Design review of the part built by this model. Coordinates are the model's own, in mm. Face numbers are marked on the shaded views. A direction names the side the tool comes from. Give positions to 0.01 mm unless a question says otherwise; leave off trailing zeros. Loops run counter-clockwise (first coordinate to the right, second up) from the corner with the lowest first, then second, coordinate; pieces in that order, holes last. Notation, with made-up numbers: M 88.25,44 L 106.25,44 A28 cw 106.25,73 Z; hole C 65.5,29.25 d11. An arc over 180 degrees is marked long. Use one line per item in the form item = value. Start each with the question number.
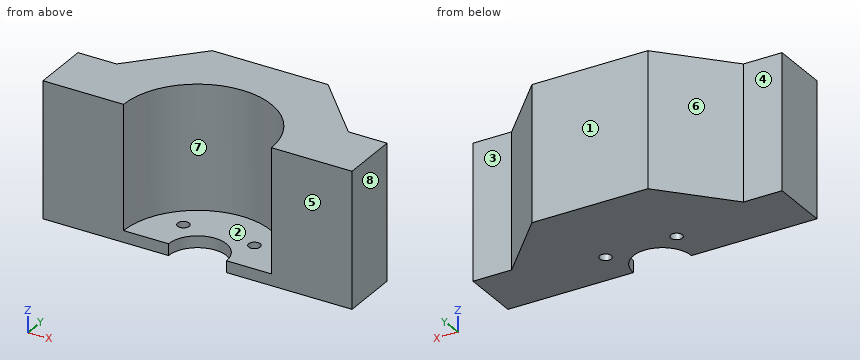
from build123d import *

# Parameters (mm, degrees)
BOSS_EXTRUDE3_DEPTH = 35
BOSS_EXTRUDE4_DEPTH = 3
SKETCH4_R           = 1.5
CUT_EXTRUDE2_DEPTH  = 4


with BuildPart() as part:
    # Sketch1 → Boss-Extrude3 (new body)
    with BuildSketch(Plane.XY):
        with BuildLine():
            Line((19.15, 0), (40, 0))
            Line((40, 0), (40, 15))
            Line((40, 15), (30, 15))
            Line((30, 15), (15, 31.15))
            Line((15, 31.15), (-15, 31.15))
            Line((-15, 31.15), (-30, 15))
            Line((-30, 15), (-40, 15))
            Line((-40, 15), (-40, 0))
            Line((-40, 0), (-19.15, 0))
            ThreePointArc((-19.15, 0), (0, 19.15), (19.15, 0))
        make_face()
    extrude(amount=BOSS_EXTRUDE3_DEPTH)

    # Sketch6 → Boss-Extrude4 (add)
    with BuildSketch(Plane(origin=(0, 0, 0), x_dir=(-1, 0, 0), z_dir=(0, 0, -1))):
        with BuildLine():
            Line((-19.15, 0), (-7.5, 0))
            ThreePointArc((-7.5, 0), (0, 7.5), (7.5, 0))
            Line((7.5, 0), (19.15, 0))
            ThreePointArc((19.15, 0), (0, 19.15), (-19.15, 0))
        make_face()
    extrude(amount=-BOSS_EXTRUDE4_DEPTH)

    # Sketch4 → Cut-Extrude2 (cut, through all)
    with BuildSketch(Plane.XY.offset(3)):
        with Locations((9.192388155, 9.192388155)):
            Circle(SKETCH4_R)
        with Locations((-9.192388155, 9.192388155)):
            Circle(SKETCH4_R)
    extrude(amount=-CUT_EXTRUDE2_DEPTH, mode=Mode.SUBTRACT)


solid = part.part
Q1. Take a section at B-B on x = 0. Give the boundary of the cut face in (y, z).
Q2. Take a section at D-D on y = 28. Give the boundary of the cut face in (x, z), plus the area to 3 significant figures.
Q3. The part is to be moulded in two halves that separate along X. For the marked faces 5, 6, 7 and 8, say which applies: pulls with the +X half, pulls with the -X half, needs draft (parallel to the pull), parting line crosses it, or undercut.
Q4. For the marked faces 1, 2, 3 and 4, list the 3-axis set-ups (+Z, -Z, +X, -X, +Y, -Y) from which the entire face can be reached by the end or side of a thin tool; tool diameter is ignored.
Q5. Take a section at C-C on y = 11.5. Give the boundary of the cut face in (x, z).
Q6. Take a section at A-A on z = 15. Give the boundary of the cut face in (x, y).
Q7. Wall thickness on probe 1 along X at (y, z) = (3, 26); probe 2 along X at (y, z) = (5.5, 31); probe 3 along Z at (x, y) = (2, 11.5): over which ranges is each line inside the solid? List them lowest first.
Q8. Clearance check with flat-ended pins moving along their axes: pin 1 Ø5 at (y, z) = (23.5, 22) entering from -X; pin 2 Ø11 at (x, z) = (-35, 11.5) entering from +Y; pin 3 Ø3 at (x, z) = (36.5, 15) entering from +Y. State where each tip first meets the part, or that it passes through.
Response values:
q1.outline = M 7.5,0 L 31.15,0 L 31.15,35 L 19.15,35 L 19.15,3 L 7.5,3 Z
q2.outline = M -17.93,0 L 17.93,0 L 17.93,35 L -17.93,35 Z
q2.area = 1,250 mm^2
q3.face_5 = needs draft
q3.face_6 = pulls with the -X half
q3.face_7 = undercut
q3.face_8 = pulls with the +X half
q4.face_1 = +Z, -Z, +X, -X, +Y
q4.face_2 = +Z, -Y
q4.face_3 = +Z, -Z, +X, +Y
q4.face_4 = +Z, -Z, -X, +Y
q5.outline = M -40,0 L 40,0 L 40,35 L 15.31,35 L 15.31,3 L -15.31,3 L -15.31,35 L -40,35 Z
q6.outline = M -40,0 L -19.15,0 A19.15 cw 19.15,0 L 40,0 L 40,15 L 30,15 L 15,31.15 L -15,31.15 L -30,15 L -40,15 Z
q7.probe_1 = -40 to -18.91, 18.91 to 40
q7.probe_2 = -40 to -18.34, 18.34 to 40
q7.probe_3 = 0 to 3
q8.pin_1 = -24.43
q8.pin_2 = 15.54
q8.pin_3 = 15
